The drawing under review shows one solid part. Ordinate dimensions are in mm from its lowest x, y, z. A direction names the side the tool comes from. Coordinates: 2 decimals unless noted, no trailing zeros. Write each loop counter-clockwise with the first axis right and the second up, starting at its lowest first coordinate (ties: lowest second). Pieces come first, ordered by that corner, then holes. Notation, with made-up numbers: (-32, 2.5) -> (-24, 2.5) arc R22 ccw to (-24, 37.5) -> close; hole circle Ø2 at (7, 46.5). An arc over 180 degrees is marked (long way). One line per question, with ' | ' between items. Start each with the question number.
Q1. For the marked faces 4 and 5, list the 3-axis set-ups (+Z, -Z, +X, -X, +Y, -Y) from which the entire face can be reached by the end or side of a thin tool; tool diameter is ignored.
Q2. Add section A-A on y = 75. State the section outline as (x, z) points, and give its area (3 significant figures).
Q3. Wall thickness on probe 1 along Y at (x, z) = (75, 14); probe 2 along Z at (x, y) = (83.5, 19); probe 3 along X at (y, z) = (85, 11.5): over which ranges is each line inside the solid? List them lowest first.
Q4. For P1, Ø4, axis at y = 65.5, z = 9.5, coming from the -X side; P2, Ø4, axis at y = 40.5, z = 4.5, coming from the +X side; P3, Ø3, axis at y = 68, z = 13, coming from the -X side, all flat-tipped, find the tip position at first contact; note any pin that passes through.
Q5. Draft analysis for pull direction Y (two halves, no side actions). For the marked faces 1, 2 and 3, state which applies: pulls with the +Y half, pulls with the -Y half, needs draft (parallel to the pull), parting line crosses it, or undercut.
Q6. Add section C-C on z = 34. State the section outline as (x, y) points (1 decimal), and give its area (3 significant figures).
Q7. Add section D-D on x = 110. State the section outline as (y, z) points.
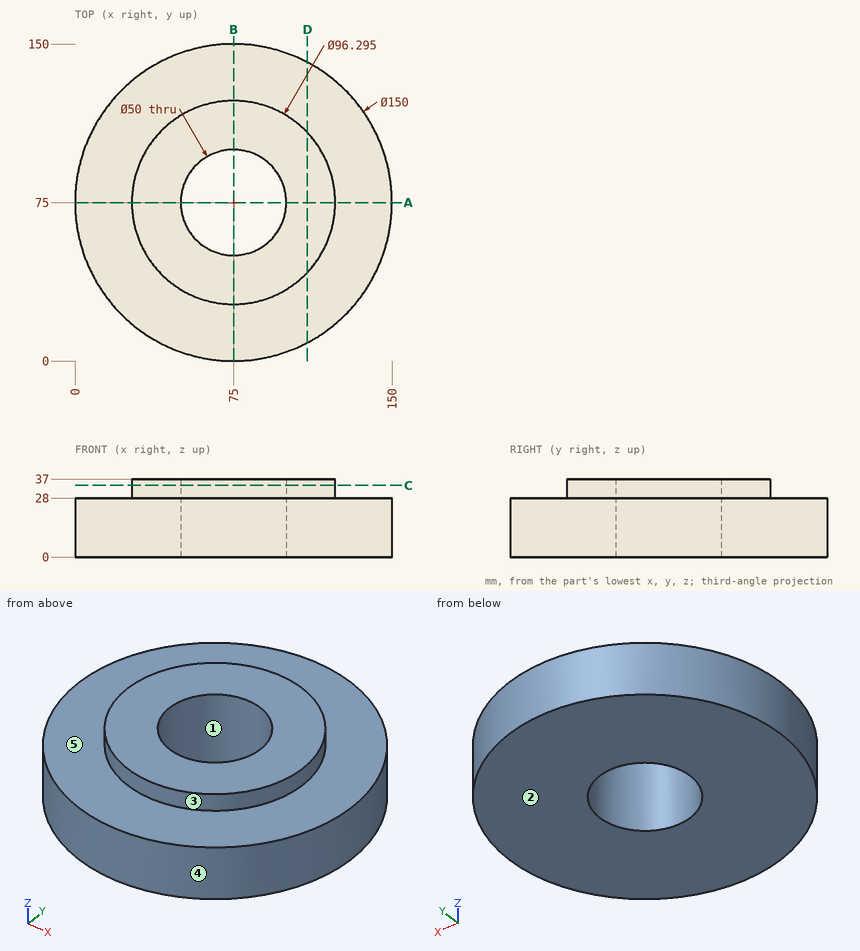
Output values:
1) face 4: +Z, -Z | face 5: +Z
2) outline: (0, 0) -> (50, 0) -> (50, 37) -> (26.85, 37) -> (26.85, 28) -> (0, 28) -> close; (100, 0) -> (150, 0) -> (150, 28) -> (123.15, 28) -> (123.15, 37) -> (100, 37) -> close | area: 3,220 mm2
3) probe 1: y = 0 to 50, 100 to 150 | probe 2: z = 0 to 28 | probe 3: x = 0.67 to 52.09, 97.91 to 149.33
4) P1: stops at x = 0.38 | P2: stops at x = 142.59 | P3: stops at x = 0.2
5) face 1: undercut | face 2: needs draft | face 3: parting line crosses it
6) outline: circle Ø96.3 at (75, 75); hole circle Ø50 at (75, 75) | area: 5,320 mm2
7) outline: (8.67, 0) -> (141.33, 0) -> (141.33, 28) -> (108.06, 28) -> (108.06, 37) -> (41.94, 37) -> (41.94, 28) -> (8.67, 28) -> close
